from build123d import *

# Parameters (mm, degrees)
SKETCH1_W                  = 914.4
SKETCH1_H                  = 711.2
BOSS_EXTRUDE1_DEPTH        = 114.3
SKETCH2_W                  = 889
SKETCH2_H                  = 685.8
CUT_EXTRUDE1_DEPTH         = 25.4
SKETCH3_W                  = 76.2
SKETCH3_H                  = 76.2
BOSS_EXTRUDE2_DEPTH        = 609.6
SKETCH4_W                  = 914.4
SKETCH4_H                  = 711.2
BOSS_EXTRUDE3_DEPTH        = 50.8
F_1_1_DIAMETER_HOLE1_D     = 25.4
F_1_1_DIAMETER_HOLE1_DEPTH = 88.9


with BuildPart() as part:
    # Sketch1 → Boss-Extrude1 (new body)
    with BuildSketch(Plane(origin=(0, 0, 0), x_dir=(1, 0, 0), z_dir=(0, 1, 0))):
        Rectangle(SKETCH1_W, SKETCH1_H)
    extrude(amount=BOSS_EXTRUDE1_DEPTH)

    # Sketch2 → Cut-Extrude1 (cut)
    with BuildSketch(Plane(origin=(0, 114.3, 0), x_dir=(1, 0, 0), z_dir=(0, 1, 0))):
        Rectangle(SKETCH2_W, SKETCH2_H)
    extrude(amount=-CUT_EXTRUDE1_DEPTH, mode=Mode.SUBTRACT)

    # Sketch3 → Boss-Extrude2 (add)
    with BuildSketch(Plane.XZ):
        with Locations((-419.1, 317.5)):
            Rectangle(SKETCH3_W, SKETCH3_H)
        with Locations((419.1, 317.5)):
            Rectangle(SKETCH3_W, SKETCH3_H)
        with Locations((419.1, -317.5)):
            Rectangle(SKETCH3_W, SKETCH3_H)
        with Locations((-419.1, -317.5)):
            Rectangle(SKETCH3_W, SKETCH3_H)
    extrude(amount=BOSS_EXTRUDE2_DEPTH)

    # Sketch4 → Boss-Extrude3 (add)
    with BuildSketch(Plane.XZ.offset(609.6)):
        Rectangle(SKETCH4_W, SKETCH4_H)
    extrude(amount=-BOSS_EXTRUDE3_DEPTH)

    # 1 (1) Diameter Hole1
    with Locations(Plane(origin=(0, 88.9, 0), x_dir=(1, 0, 0), z_dir=(0, 1, 0))):
        with Locations((-274.028125044, 34.29999998), (274.028125044, 34.29999998)):
            Hole(F_1_1_DIAMETER_HOLE1_D / 2, depth=F_1_1_DIAMETER_HOLE1_DEPTH)


solid = part.part
Build history of the part. All positions in model axes, mm. A direction names the side the tool comes from. Give positions to 0.01 mm unless a question says otherwise; leave off trailing zeros. Order: outer loops, then holes, each group sorted by start corner. A loop starts at its lowest first (then second) coordinate and runs counter-clockwise, first axis right, second up. Notation, with made-up numbers: M 89.5,75 L 112.5,75 A18 cw 112.5,108 Z; hole C 43,-16 d3. An arc over 180 degrees is marked long. Use one line per item in the form item = value.
Q1. Wall check: probe 1 along X at (y, z) = (61, -34); probe 2 along X at (y, z) = (-279.5, -291); probe 3 along Y at (x, z) = (263.5, 128.5). Give the ranges that are in metal, low to high.
Conclusion:
probe_1 = -457.2 to -286.72, -261.33 to 261.33, 286.72 to 457.2
probe_2 = -457.2 to -381, 381 to 457.2
probe_3 = -609.6 to -558.8, 0 to 88.9
Q2. Pin check, flat tips, straight feed: P1, Ø1, axis at x = -17, z = 269, coming from the +Y side; P2, Ø23, axis at x = -274.03, z = -34.3, coming from the +Y side. Stop position of each tip, or through.
Conclusion:
P1 = 88.9
P2 = -558.8
Q3. Pull direction Y, two halves, no side cores. Call faces 4 (the flat face through (-420, -275, -279.4)), 5 (the flat face through (-6, -609.6, 5)), 6 (the flat face through (-6, 0, -5)), 7 (the flat face through (457.2, -253, 311)): released by +Y, released by -Y, zero draft, split by the parting line, or undercut.
Conclusion:
face_4 = undercut
face_5 = released by -Y
face_6 = undercut
face_7 = zero draft
Q4. Which spindle directions (+Z, -Z, +X, -X, +Y, -Y) get a long thin tool onto all of the face, cutting with end or side? Do faces 1 (the flat face through (381, -275, 317)), 2 (the flat face through (-6, -558.8, 5)), 3 (the flat face through (-420, -275, 279.4)). Say none if no direction does.
Conclusion:
face_1 = +Z, -Z
face_2 = none
face_3 = +X, -X
Q5. Slice it at B-B, the plane z = -34.3. Write the cut outline in (x, y), and give its area (3 significant figures).
Conclusion:
outline = M -457.2,-609.6 L 457.2,-609.6 L 457.2,-558.8 L -457.2,-558.8 Z; M -457.2,0 L -286.73,0 L -286.73,88.9 L -444.5,88.9 L -444.5,114.3 L -457.2,114.3 Z; M -261.33,0 L 261.33,0 L 261.33,88.9 L -261.33,88.9 Z; M 286.73,0 L 457.2,0 L 457.2,114.3 L 444.5,114.3 L 444.5,88.9 L 286.73,88.9 Z
area = 124,000 mm2
Q6. Slice it at C-C, the plane x = 227. Write the cut outline in (y, z), and give its area (4 significant figures).
Conclusion:
outline = M -609.6,-355.6 L -558.8,-355.6 L -558.8,355.6 L -609.6,355.6 Z; M 0,-355.6 L 114.3,-355.6 L 114.3,-342.9 L 88.9,-342.9 L 88.9,342.9 L 114.3,342.9 L 114.3,355.6 L 0,355.6 Z
area = 100,000 mm2
Q7. Slice it at A-A, the plane y = -511. Write the cut outline in (x, z).
Conclusion:
outline = M -457.2,-355.6 L -381,-355.6 L -381,-279.4 L -457.2,-279.4 Z; M -457.2,279.4 L -381,279.4 L -381,355.6 L -457.2,355.6 Z; M 381,-355.6 L 457.2,-355.6 L 457.2,-279.4 L 381,-279.4 Z; M 381,279.4 L 457.2,279.4 L 457.2,355.6 L 381,355.6 Z
